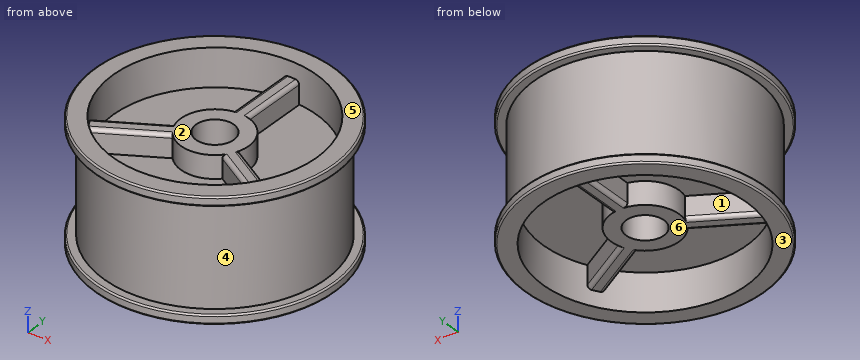
from build123d import *

# Parameters (mm, degrees)
SKETCH4_R           = 12.5
BOSS_EXTRUDE1_DEPTH = 30
SKETCH6_R           = 12.5
CUT_EXTRUDE1_DEPTH  = 71
FILLET1_R           = 2.5
SCALE1_SCALE        = 0.5


with BuildPart() as part:
    # Sketch3 → Revolve1 (revolve)
    with BuildSketch(Plane(origin=(0, 0, 0), x_dir=(0, 0, -1), z_dir=(1, 0, 0))):
        with BuildLine():
            Line((-40, 158.392005271), (-40, 147.392005271))
            Line((-40, 147.392005271), (-15, 147.392005271))
            Line((-15, 147.392005271), (-15, 80))
            Line((-15, 80), (0, 80))
            Line((0, 80), (15, 80))
            Line((15, 80), (15, 147.392005271))
            Line((15, 147.392005271), (40, 147.392005271))
            Line((40, 147.392005271), (40, 158.392005271))
            ThreePointArc((40, 158.392005271), (39.707106781, 159.099112052), (39, 159.392005271))
            Line((39, 159.392005271), (35, 159.392005271))
            ThreePointArc((35, 159.392005271), (34.292893219, 159.099112052), (34, 158.392005271))
            Line((34, 158.392005271), (34, 153.392005271))
            Line((34, 153.392005271), (-34, 153.392005271))
            Line((-34, 153.392005271), (-34, 158.392005271))
            ThreePointArc((-34, 158.392005271), (-34.292893219, 159.099112052), (-35, 159.392005271))
            Line((-35, 159.392005271), (-39, 159.392005271))
            ThreePointArc((-39, 159.392005271), (-39.707106781, 159.099112052), (-40, 158.392005271))
        make_face()
    revolve(axis=Axis((0, 80, 0), (0, 0, 1)))

    # Sketch4 → Boss-Extrude1 (add, symmetric)
    with BuildSketch(Plane.XY):
        with BuildLine():
            Line((-5, 101.937410968), (-5, 146.922350015))
            ThreePointArc((-5, 146.922350015), (0, 147.108873716), (5, 146.922350015))
            Line((5, 146.922350015), (5, 101.937410968))
            ThreePointArc((5, 101.937410968), (19.485571585, 91.25), (21.498355192, 73.361421535))
            Line((21.498355192, 73.361421535), (60.456455194, 50.868952012))
            ThreePointArc((60.456455194, 50.868952012), (58.117989458, 46.445563142), (55.456455194, 42.208697974))
            Line((55.456455194, 42.208697974), (16.498355192, 64.701167497))
            ThreePointArc((16.498355192, 64.701167497), (0, 57.5), (-16.498355192, 64.701167497))
            Line((-16.498355192, 64.701167497), (-55.456455194, 42.208697974))
            ThreePointArc((-55.456455194, 42.208697974), (-58.117989458, 46.445563142), (-60.456455194, 50.868952012))
            Line((-60.456455194, 50.868952012), (-21.498355192, 73.361421535))
            ThreePointArc((-21.498355192, 73.361421535), (-19.485571585, 91.25), (-5, 101.937410968))
        make_face()
        with Locations((0, 80)):
            Circle(SKETCH4_R, mode=Mode.SUBTRACT)
    extrude(amount=BOSS_EXTRUDE1_DEPTH, both=True)

    # Sketch6 → Cut-Extrude1 (cut, through all)
    with BuildSketch(Plane.XY.offset(30)):
        with Locations((0, 80)):
            Circle(SKETCH6_R)
    extrude(amount=-CUT_EXTRUDE1_DEPTH, mode=Mode.SUBTRACT)

    # Fillet1
    fillet1_edges = [part.edges().sort_by_distance(p)[0] for p in [
        (-40.977405193, 62.115186773, -30),
        (-35.977405193, 53.454932735, -30),
        (35.977405193, 53.454932735, -30),
        (40.977405193, 62.115186773, -30),
        (5, 124.429880492, -30),
        (-5, 124.429880492, -30),
        (-40.977405193, 62.115186773, 30),
        (-35.977405193, 53.454932735, 30),
        (35.977405193, 53.454932735, 30),
        (40.977405193, 62.115186773, 30),
        (5, 124.429880492, 30),
        (-5, 124.429880492, 30),
    ]]
    fillet(fillet1_edges, radius=FILLET1_R)


with BuildPart() as part_1:
    # Scale1: scaled about (-4.6e-08, 79.999999971, -2.91e-07)
    add(part.part.scale(SCALE1_SCALE).moved(Location((-2.3e-08, 39.999999985, -1.45e-07))))


solid = part_1.part
The model under review builds one solid part; all positions refer to its coordinate system, in mm. Face numbers are marked on the shaded views. A direction names the side the tool comes from. Round coordinates to 2 decimals unless told otherwise and drop trailing zeros. Loops run counter-clockwise (first coordinate to the right, second up) from the corner with the lowest first, then second, coordinate; pieces in that order, holes last. Notation, with made-up numbers: (-6.5, 24) -> (44.5, 24) arc R31 cw to (44.5, 51) -> close; hole circle Ø9 at (29, -14.75). An arc over 180 degrees is marked (long way). Answer as CSV lines item,"result".
1) Draft analysis for pull direction Y (two halves, no side actions). For the marked faces 4, 5 and 6, state which applies: pulls with the +Y half, pulls with the -Y half, needs draft (parallel to the pull), parting line crosses it, or undercut.
Geometry results:
face 4,"parting line crosses it"
face 5,"needs draft"
face 6,"undercut"
2) Tool access review of the marked faces 1, 2 and 3: name each direction out of +Z, -Z, +X, -X, +Y, -Y from which nothing blocks a thin tool from reaching the whole face with its end or side.
Geometry results:
face 1,"-Z"
face 2,"+Z"
face 3,"-Z, +X, -X, +Y, -Y"
3) Add section A-A on z = 11.5. Write out the cut boundary in (x, y).
Geometry results:
outline,"circle Ø73.39 at (0, 80); (-30.23, 65.43) arc R33.55 ccw to (-27.73, 61.1) -> (-8.25, 72.35) arc R11.25 ccw to (8.25, 72.35) -> (27.73, 61.1) arc R33.55 ccw to (30.23, 65.43) -> (10.75, 76.68) arc R11.25 ccw to (2.5, 90.97) -> (2.5, 113.46) arc R33.55 ccw to (-2.5, 113.46) -> (-2.5, 90.97) arc R11.25 ccw to (-10.75, 76.68) -> close; hole circle Ø67.39 at (0, 80); hole circle Ø12.5 at (0, 80)"
4) For P1, Ø6, axis at y = 100, z = -9.5, coming from the -X side; P2, Ø5, axis at y = 105, z = -10.5, coming from the -X side; P3, Ø3, axis at y = 90, z = -15, coming from the -X side, all flat-tipped, find the tip position at first contact; note any pin that passes through.
Geometry results:
P1,"stops at x = -32.52"
P2,"stops at x = -28.99"
P3,"stops at x = -35.7"
5) Add section C-C on z = 16. Write out the cut boundary in (x, y), plus the area to 3 significant figures.
Geometry results:
outline,"circle Ø73.39 at (0, 80); hole circle Ø67.39 at (0, 80)"
area,"663 mm²"
6) Add section B-B on z = -4.5. Write out the cut boundary in (x, y), plus the area to 3 significant figures.
Geometry results:
outline,"circle Ø73.39 at (0, 80); hole circle Ø12.5 at (0, 80)"
area,"4,110 mm²"
7) To check wall thickness, follow line 1 along X through (y, z) = (80, 11); line 2 along Y through (x, z) = (-24, 8.5); line 3 along X through (y, z) = (80, -6.25). State the ranges of each line that lie inside material, in increasing order. Write a range as from..to.
Geometry results:
line 1,"x = -36.7..-33.7, -11.25..-6.25, 6.25..11.25, 33.7..36.7"
line 2,"y = 52.24..56.35, 63.26..69.03, 103.65..107.76"
line 3,"x = -36.7..-6.25, 6.25..36.7"
